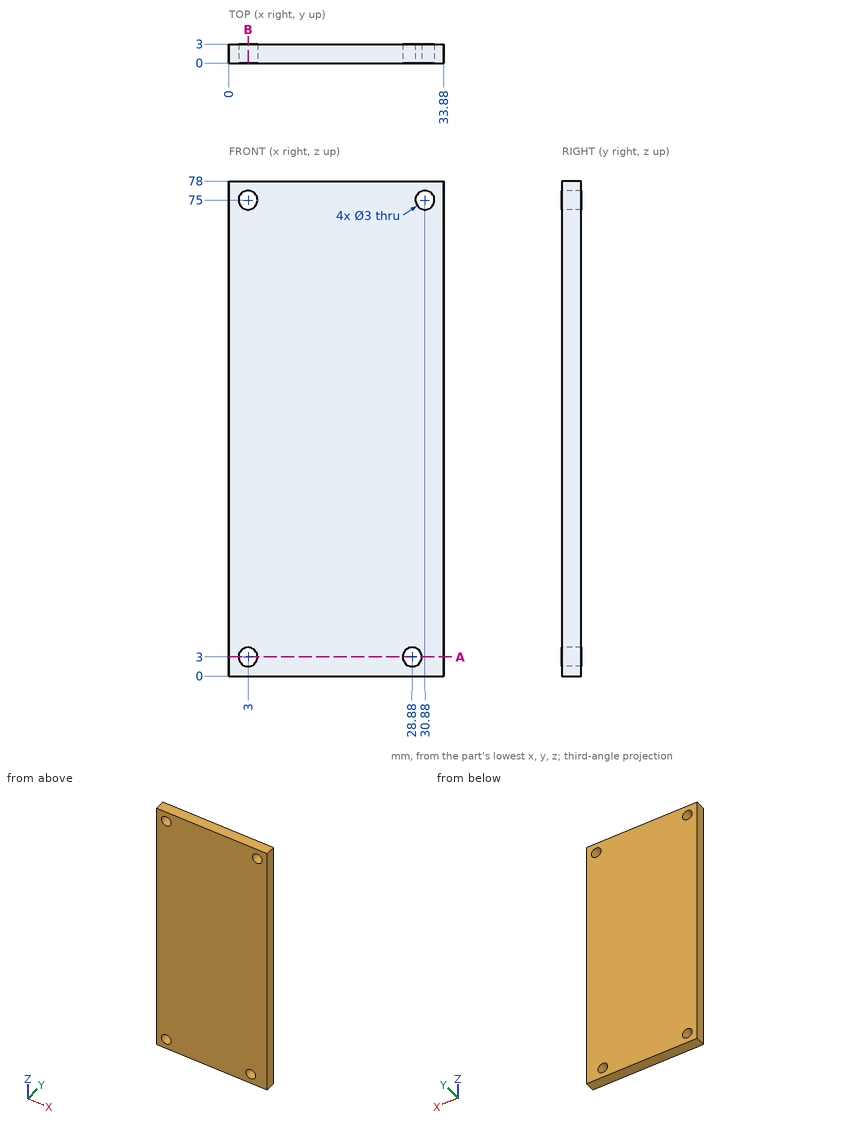
Part print with two shaded views. Sizes in mm from the minimum x, y, z corner. Coordinates: 2 decimals unless noted, no trailing zeros. Order: outer loops, then holes, each group sorted by start corner. A loop starts at its lowest first (then second) coordinate and runs counter-clockwise, first axis right, second up. Notation, with made-up numbers: M -20.75,76 L 8.25,76 A29 ccw 8.25,112 Z; hole C -32.5,-38.75 d2. An arc over 180 degrees is marked long. One line per question, with ' | ' between items. Start each with the question number.
1. Cut at B-B (x = 3). Write the cut outline in (y, z).
2. Cut at A-A (z = 3). Write the cut outline in (x, y), plus the area to 3 significant figures.
3. Wall check: line 1 along Z through (x, y) = (3, 1.9); line 2 along X through (y, z) = (1.3, 3); line 3 along X through (y, z) = (2.4, 75). Give the ranges that are in metal, low to high. Write a range as [from, to].
The answers:
1) outline: M 0,0 L 3,0 L 3,1.5 L 0,1.5 Z; M 0,4.5 L 3,4.5 L 3,73.5 L 0,73.5 Z; M 0,76.5 L 3,76.5 L 3,78 L 0,78 Z
2) outline: M 0,0 L 1.5,0 L 1.5,3 L 0,3 Z; M 4.5,0 L 27.38,0 L 27.38,3 L 4.5,3 Z; M 30.38,0 L 33.88,0 L 33.88,3 L 30.38,3 Z | area: 83.6 mm2
3) line 1: z = [0, 1.5], [4.5, 73.5], [76.5, 78] | line 2: x = [0, 1.5], [4.5, 27.38], [30.38, 33.88] | line 3: x = [0, 1.5], [4.5, 29.38], [32.38, 33.88]
